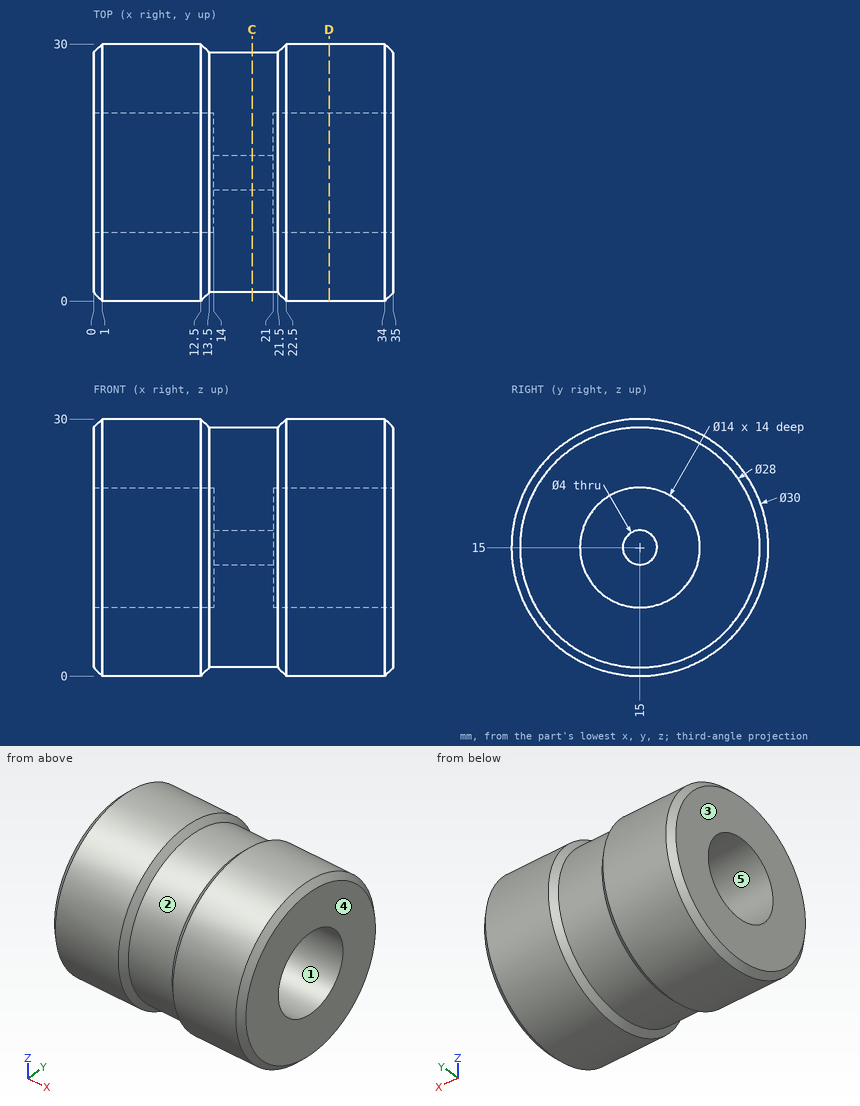
Part print with two shaded views. Sizes in mm from the minimum x, y, z corner. A direction names the side the tool comes from. Round coordinates to 2 decimals unless told otherwise and drop trailing zeros. Loops run counter-clockwise (first coordinate to the right, second up) from the corner with the lowest first, then second, coordinate; pieces in that order, holes last.
Item 1: Two-plate mould, pull along Y, no slides. Class the marked faces 1, 2 and 3: released by +Y, released by -Y, zero draft, split by the parting line, or undercut.
Item 2: Which spindle directions (+Z, -Z, +X, -X, +Y, -Y) get a long thin tool onto all of the face, cutting with end or side? Do the marked faces 4 and 5. Say none if no direction does.
Item 3: Saw through at D-D (x = 27.5). List the corners of the cut face in (y, z).
Item 4: Pin check, flat tips, straight feed: P1, Ø4, axis at x = 21, y = 10.5, coming from the -Z side; P2, Ø3, axis at x = 23, y = 5.5, coming from the +Z side; P3, Ø1, axis at x = 5.5, y = 21, coming from the +Z side (1 decimal). Stop position of each tip, or through.
Item 5: Drill centre lines: line 1 along Y through (x, z) = (3, 15); line 2 along Y through (x, z) = (23, 10.75) (1 decimal); line 3 along Z through (x, y) = (22, 15.5). Where is each one in solid material? Low to high.
Item 6: Saw through at C-C (x = 18.5). List the corners of the cut face in (y, z), then the cut area to 3 significant figures.
Worked answers:
1. face 1: undercut
1. face 2: split by the parting line
1. face 3: zero draft
2. face 4: +Z, -Z, +X, +Y, -Y
2. face 5: -X
3. outline: circle Ø30 at (15, 15); hole circle Ø14 at (15, 15)
4. P1: stops at z = 0.34
4. P2: stops at z = 27.69
4. P3: stops at z = 29
5. line 1: y = 0 to 8, 22 to 30
5. line 2: y = 0.6 to 9.4, 20.6 to 29.4
5. line 3: z = 0.51 to 8.02, 21.98 to 29.49
6. outline: circle Ø28 at (15, 15); hole circle Ø4 at (15, 15)
6. area: 603 mm2
